from build123d import *

# Parameters (mm, degrees)
SKETCH_1_R          = 25
SKETCH_1_R_2        = 20
EXTRUDE_1_DEPTH     = 80
SKETCH_2_W          = 5
SKETCH_2_H          = 4
CUT_EXTRUDE_1_DEPTH = 80


with BuildPart() as part:
    # Эскиз1 → Бобышка-Вытянуть1 (new body)
    with BuildSketch(Plane(origin=(0, 0, 0), x_dir=(0, 0, -1), z_dir=(1, 0, 0))):
        Circle(SKETCH_1_R)
        Circle(SKETCH_1_R_2, mode=Mode.SUBTRACT)
    extrude(amount=EXTRUDE_1_DEPTH)

    # Эскиз2 → Вырез-Вытянуть1 (cut)
    with BuildSketch(Plane.XY):
        with Locations((2.5, 0)):
            Rectangle(SKETCH_2_W, SKETCH_2_H)
    extrude(amount=-CUT_EXTRUDE_1_DEPTH, mode=Mode.SUBTRACT)


solid = part.part
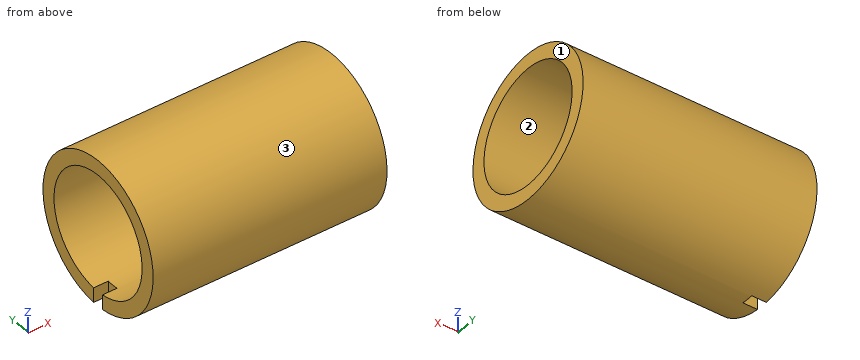
Geometry: final body of the model. Coordinates: model frame, mm. Face numbers are marked on the shaded views. Give positions to 0.01 mm unless a question says otherwise; leave off trailing zeros. Order: outer loops, then holes, each group sorted by start corner. A loop starts at its lowest first (then second) coordinate and runs counter-clockwise, first axis right, second up. Notation, with made-up numbers: (-6.75, 7.5) -> (21.25, 7.5) arc R19 cw to (21.25, 12.5) -> close; hole circle Ø7 at (34.25, -25.5). An arc over 180 degrees is marked (long way). Answer as a JSON object with one key per item and string values.
Q1. Draft query along Z for the marked faces 1, 2 and 3. Return one class per face: released by +Z, released by -Z, zero draft, split by the parting line, or undercut.
Entries:
{"face 1": "zero draft", "face 2": "undercut", "face 3": "split by the parting line"}
Q2. First-contact query: pin 1 (12 mm diameter, centred on x = 63, y = -20, fed in from -Z); pin 2 (1.5 mm diameter, centred on x = 48.5, z = -8, fed in from -Y); pin 3 (5 mm diameter, centred on x = 29, z = -12, fed in from +Y); pin 4 (8 mm diameter, centred on y = 11.5, z = 3.5, fed in from -X). Flat tips, straight axial feed; report the tip coordinate or a pass-through.
Entries:
{"pin 1": "stops at z = -20.71", "pin 2": "stops at y = -23.93", "pin 3": "stops at y = 23.12", "pin 4": "passes through"}
Q3. Section A-A (z = 0). Output: boundary loops of the cut face in (x, y).
Entries:
{"outline": "(0, -25) -> (80, -25) -> (80, -20) -> (0, -20) -> close; (0, 20) -> (80, 20) -> (80, 25) -> (0, 25) -> close"}
Q4. Section B-B (y = 0). Output: boundary loops of the cut face in (x, z), plus the area to 3 significant figures.
Entries:
{"outline": "(0, 20) -> (80, 20) -> (80, 25) -> (0, 25) -> close; (5, -25) -> (80, -25) -> (80, -20) -> (5, -20) -> close", "area": "775 mm^2"}
Q5. Section C-C (x = 54.5). Output: boundary loops of the cut face in (y, z), plus the area to 3 significant figures.
Entries:
{"outline": "circle Ø50 at (0, 0); hole circle Ø40 at (0, 0)", "area": "707 mm^2"}
Q6. Material intervals for probe 1 along Z at (x, y) = (49, 0); probe 2 along Z at (x, y) = (31, 18), sorted ascending.
Entries:
{"probe 1": "z = -25 to -20, 20 to 25", "probe 2": "z = -17.35 to -8.72, 8.72 to 17.35"}
